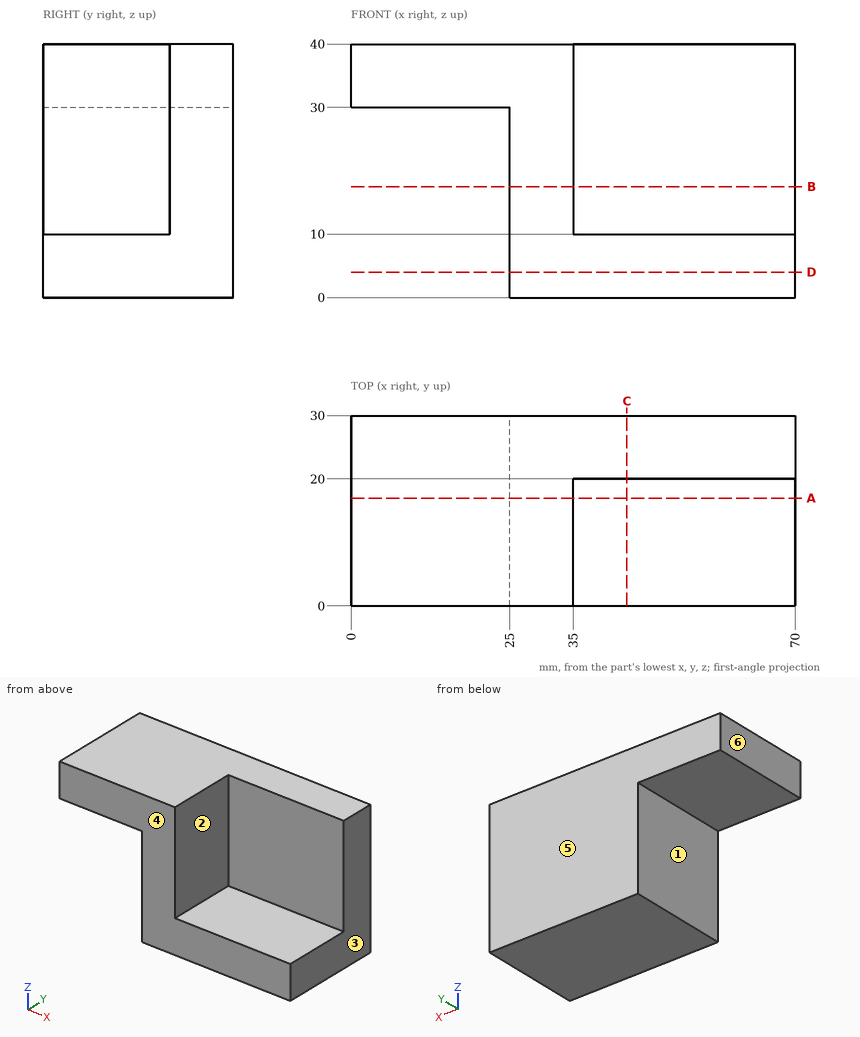
Part print with two shaded views. Sizes in mm from the minimum x, y, z corner. A direction names the side the tool comes from. Round coordinates to 2 decimals unless told otherwise and drop trailing zeros. Order: outer loops, then holes, each group sorted by start corner. A loop starts at its lowest first (then second) coordinate and runs counter-clockwise, first axis right, second up. Notation, with made-up numbers: (48.5, 43.25) -> (71.5, 43.25) arc R12 cw to (71.5, 59.25) -> close; hole circle Ø1 at (6.25, 31.5). An arc over 180 degrees is marked (long way). Write each question's results on one line, items separated by ' | '.
1. Cut at B-B (z = 17.5). Give the cut face in (x, y).
Findings below:
outline: (25, 0) -> (35, 0) -> (35, 20) -> (70, 20) -> (70, 30) -> (25, 30) -> close
2. Cut at C-C (x = 43.5). Give the cut face in (y, z).
Findings below:
outline: (0, 0) -> (30, 0) -> (30, 40) -> (20, 40) -> (20, 10) -> (0, 10) -> close
3. 3-axis set-ups, long thin cutter, end or side, ignore diameter. For the marked faces 1, 2 and 3: which of +Z, -Z, +X, -X, +Y, -Y reach the whole face in a straight line?
Findings below:
face 1: -Z, -X, +Y, -Y | face 2: +Z, +X, -Y | face 3: +Z, -Z, +X, +Y, -Y
4. Pull direction Y, two halves, no side cores. Call the marked faces 4, 5 and 6: pulls with the +Y half, pulls with the -Y half, needs draft (parallel to the pull), parting line crosses it, or undercut.
Findings below:
face 4: pulls with the -Y half | face 5: pulls with the +Y half | face 6: needs draft
5. Wall check: line 1 along Y through (x, z) = (61, 28.5); line 2 along X through (y, z) = (1.5, 12); line 3 along Z through (x, y) = (24, 9.5). Give the ranges that are in metal, low to high. Write a range as [from, to].
Findings below:
line 1: y = [20, 30] | line 2: x = [25, 35] | line 3: z = [30, 40]
6. Cut at A-A (y = 17). Give the cut face in (x, z).
Findings below:
outline: (0, 30) -> (25, 30) -> (25, 0) -> (70, 0) -> (70, 10) -> (35, 10) -> (35, 40) -> (0, 40) -> close
7. Flat gauge pins, fed straight in: P1, Ø12, axis at x = 53.5, z = 22, coming from the -Y side; P2, Ø5, axis at y = 10, z = 18.5, coming from the -X side; P3, Ø16, axis at x = 44.5, y = 7.5, coming from the +Z side. Where does each tip first touch, or does it go through?
Findings below:
P1: stops at y = 20 | P2: stops at x = 25 | P3: stops at z = 10
8. Cut at D-D (z = 4). Give the cut face in (x, y), plus the area to 3 significant figures.
Findings below:
outline: (25, 0) -> (70, 0) -> (70, 30) -> (25, 30) -> close | area: 1,350 mm²
